```python
from build123d import *

# Parameters (mm, degrees)
MODEL_R         = 1.5999968
MODEL_R_2       = 2.0999958
MODEL_R_3       = 11.499977
EXTRUDE_1_DEPTH = 4
EXTRUDE_2_DEPTH = 4
FILLET_1_R      = 5
SKETCH_2_R      = 2.1
EXTRUDE_3_DEPTH = 4
EXTRUDE_4_DEPTH = 4


with BuildPart() as part:
    # Model → Бобышка-Вытянуть1 (new body)
    with BuildSketch(Plane.XY):
        with BuildLine():
            Line((274.028195208, 189.164211852), (274.028195208, 151.235355522))
            ThreePointArc((274.028195208, 151.235355522), (273.647593631, 149.321942187), (272.563732042, 147.699828687))
            Line((272.563732042, 147.699828687), (265.492678373, 140.628775017))
            ThreePointArc((265.492678373, 140.628775017), (264.408816784, 139.006661518), (264.028215208, 137.093248183))
            Line((264.028215208, 137.093248183), (264.028215208, 124.164341852))
            ThreePointArc((264.028215208, 124.164341852), (262.563752042, 120.628815017), (259.028225208, 119.164351852))
            Line((259.028225208, 119.164351852), (249.028245208, 119.164351852))
            ThreePointArc((249.028245208, 119.164351852), (245.492718373, 117.699888687), (244.028255208, 114.164361852))
            Line((244.028255208, 114.164361852), (244.028255208, 104.164381852))
            ThreePointArc((244.028255208, 104.164381852), (242.563792042, 100.628855017), (239.028265208, 99.164391852))
            Line((239.028265208, 99.164391852), (229.028285208, 99.164391852))
            ThreePointArc((229.028285208, 99.164391852), (225.492758373, 100.628855017), (224.028295208, 104.164381852))
            Line((224.028295208, 104.164381852), (224.028295208, 189.164211852))
            ThreePointArc((224.028295208, 189.164211852), (225.492758373, 192.699738687), (229.028285208, 194.164201852))
            Line((229.028285208, 194.164201852), (269.028205208, 194.164201852))
            ThreePointArc((269.028205208, 194.164201852), (272.563732043, 192.699738687), (274.028195208, 189.164211852))
        make_face()
        with Locations((267.528208208, 184.664220852)):
            Circle(MODEL_R, mode=Mode.SUBTRACT)
        with Locations((267.528208208, 153.664282852)):
            Circle(MODEL_R, mode=Mode.SUBTRACT)
        with Locations((236.528270208, 153.664282852)):
            Circle(MODEL_R, mode=Mode.SUBTRACT)
        with Locations((236.528270208, 184.664220852)):
            Circle(MODEL_R, mode=Mode.SUBTRACT)
        with Locations((254.028235208, 127.164335852)):
            Circle(MODEL_R_2, mode=Mode.SUBTRACT)
        with Locations((234.028275208, 127.164335852)):
            Circle(MODEL_R_2, mode=Mode.SUBTRACT)
        with Locations((234.028275208, 109.164371852)):
            Circle(MODEL_R_2, mode=Mode.SUBTRACT)
        with Locations((252.028239208, 169.164251852)):
            Circle(MODEL_R_3, mode=Mode.SUBTRACT)
    extrude(amount=EXTRUDE_1_DEPTH)

    # Эскиз1 → Бобышка-Вытянуть2 (add)
    with BuildSketch(Plane(origin=(0, 0, 0), x_dir=(-1, 0, 0), z_dir=(0, 0, -1))):
        Polygon((-274.028195208, 194.164201852), (-286.028195208, 194.164201852), (-286.028195208, 147.699828687), (-274.028195208, 147.699828687), (-271.528200208, 147.699828687), (-271.528200208, 152.064286052), (-274.028195208, 152.064286052), (-274.028195208, 189.164211852), (-269.028205208, 189.164211852), (-269.028205208, 194.164201852), align=None)
    extrude(amount=-EXTRUDE_2_DEPTH)

    # Скругление1
    fillet_1_edges = [part.edges().sort_by_distance(p)[0] for p in [
        (272.563732042, 147.699828687, 2),
    ]]
    fillet(fillet_1_edges, radius=FILLET_1_R)

    # Эскиз2 → Бобышка-Вытянуть3 (add)
    with BuildSketch(Plane(origin=(286.028195208, 0, 0), x_dir=(0, 0, -1), z_dir=(1, 0, 0))):
        with BuildLine():
            Line((0, 147.699828687), (-40, 147.699828687))
            ThreePointArc((-40, 147.699828687), (-43.535533906, 149.164294781), (-45, 152.699828687))
            Line((-45, 152.699828687), (-45, 189.164201852))
            ThreePointArc((-45, 189.164201852), (-43.535533906, 192.699735758), (-40, 194.164201852))
            Line((-40, 194.164201852), (0, 194.164201852))
            Line((0, 194.164201852), (0, 147.699828687))
        make_face()
        with Locations((-40, 189.164201852)):
            Circle(SKETCH_2_R, mode=Mode.SUBTRACT)
        with Locations((-40, 152.699828687)):
            Circle(SKETCH_2_R, mode=Mode.SUBTRACT)
        with Locations((-20, 189.164201852)):
            Circle(SKETCH_2_R, mode=Mode.SUBTRACT)
        with Locations((-20, 152.699828687)):
            Circle(SKETCH_2_R, mode=Mode.SUBTRACT)
    extrude(amount=EXTRUDE_3_DEPTH)

    # Эскиз3 → Бобышка-Вытянуть4 (add)
    with BuildSketch(Plane(origin=(0, 194.164201852, 0), x_dir=(1, 0, 0), z_dir=(0, 1, 0))):
        Polygon((286.028195208, -4), (276.028195208, -4), (286.028195208, -14), align=None)
    extrude_4 = extrude(amount=-EXTRUDE_4_DEPTH)

    # Зеркальное отражение1: Бобышка-Вытянуть4 across plane
    add(extrude_4.mirror(Plane.ZX.offset(170.93201527)))


solid = part.part
```
Build history of the part. All positions in model axes, mm. A direction names the side the tool comes from. Give positions to 0.01 mm unless a question says otherwise; leave off trailing zeros. Loops run counter-clockwise (first coordinate to the right, second up) from the corner with the lowest first, then second, coordinate; pieces in that order, holes last.
1) Band-saw the part on C-C on z = 29. List the corners of the cut face in (x, y).
Values follow:
outline: (286.03, 147.7) - (290.03, 147.7) - (290.03, 194.16) - (286.03, 194.16) - close
2) Drop flat-ended pins along their axis: P1, Ø6.5, axis at y = 152.7, z = 40, coming from the -X side; P2, Ø2, axis at y = 128, z = 1.5, coming from the +X side; P3, Ø3, axis at x = 256, z = 2.5, coming from the -Y side. Give the stop position or say it passes through.
Values follow:
P1: stops at x = 286.03
P2: stops at x = 264.03
P3: stops at y = 119.16
3) 3-axis set-ups, long thin cutter, end or side, ignore diameter. For faces 5 (the face through (290.028, 171, 22)), 6 (the face through (248.6, 157.9, 4)), 7 (the face through (244.028, 109, 2)): which of +Z, -Z, +X, -X, +Y, -Y reach the whole face in a straight line?
Values follow:
face 5: +Z, -Z, +X, +Y, -Y
face 6: +Z, -X
face 7: +Z, -Z, +X, -Y
4) Band-saw the part on B-B on x = 250.5. List the corners of the cut face in (y, z).
Values follow:
outline: (119.16, 0) - (157.77, 0) - (157.77, 4) - (119.16, 4) - close; (180.56, 0) - (194.16, 0) - (194.16, 4) - (180.56, 4) - close
5) Probe line 1 along Y through (x, z) = (288.75, 20); line 2 along Z through (x, y) = (259.5, 124); line 3 along X through (y, z) = (179, 14). List the from-to ranges inside material, lowest first.
Values follow:
line 1: y = 147.7 to 150.6, 154.8 to 187.06, 191.26 to 194.16
line 2: z = 0 to 4
line 3: x = 286.03 to 290.03
6) Band-saw the part on A-A on z = 20. List the corners of the cut face in (x, y), then the cut area to 3 significant figures.
Values follow:
outline: (286.03, 147.7) - (290.03, 147.7) - (290.03, 150.6) - (286.03, 150.6) - close; (286.03, 154.8) - (290.03, 154.8) - (290.03, 187.06) - (286.03, 187.06) - close; (286.03, 191.26) - (290.03, 191.26) - (290.03, 194.16) - (286.03, 194.16) - close
area: 152 mm2
7) Two-plate mould, pull along X, no slides. Class faces 1 (the face through (225.454, 192.661, 1.972)), 2 (the face through (268.267, 152.245, 1.972)), 3 (the face through (236.32, 186.25, 1.97)), 4 (the face through (272.7, 147.31, 2.03)): released by +X, released by -X, zero draft, split by the parting line, or undercut.
Values follow:
face 1: released by -X
face 2: undercut
face 3: undercut
face 4: released by +X
